Build history of the part. All positions in model axes, mm. A direction names the side the tool comes from. Round coordinates to 2 decimals unless told otherwise and drop trailing zeros. Order: outer loops, then holes, each group sorted by start corner. A loop starts at its lowest first (then second) coordinate and runs counter-clockwise, first axis right, second up. Notation, with made-up numbers: (21.5, 6) -> (47.5, 6) arc R9 cw to (47.5, 12) -> close; hole circle Ø6 at (31.25, 25.25). An arc over 180 degrees is marked (long way). Use a Markdown table: item, result. Add a question column.
Item 1: Two-plate mould, pull along X, no slides. Class faces 1 (the face through (59, 25, 18)), 2 (the face through (0, 0, 29)), 3 (the face through (69.14, 24.65, -29.1)): released by +X, released by -X, zero draft, split by the parting line, or undercut.
Item 2: Probe L1, parallel to Z at x = 42.5, y = 31; L2, parallel to X at y = 13.5, z = -10.5; L3, parallel to X at y = 19, z = -24. List the from-to ranges inside material, lowest first.
Item 3: Slice it at C-C, the plane z = -0.5. Give the cut face in (x, y), plus the area to 3 significant figures.
Item 4: Slice it at A-A, the plane x = 21. Give the cut face in (y, z).
Item 5: Slice it at B-B, the plane x = -60. Give the cut face in (y, z).
Item 6: 3-axis set-ups, long thin cutter, end or side, ignore diameter. For faces 4 (the face through (69.26, 15.726, 2.059)), 5 (the face through (67.74, 11.82, -2.93)), 6 (the face through (-60, 25, 18)): which of +Z, -Z, +X, -X, +Y, -Y reach the whole face in a straight line?
Item 7: Slice it at D-D, the plane y = 25. State how many separate pieces and enclosed holes the cut face has, plus the area to 3 significant figures.
from build123d import *

# Parameters (mm, degrees)
SKETCH1_R           = 2.75
SKETCH1_W           = 130
SKETCH1_H           = 38
BOSS_EXTRUDE1_DEPTH = 10
SKETCH1_2_W         = 130
SKETCH1_2_H         = 38
BOSS_EXTRUDE2_DEPTH = 10
SKETCH14_W          = 15
SKETCH14_H          = 36
SKETCH14_W_2        = 104
SKETCH14_H_2        = 9
CUT_EXTRUDE2_DEPTH  = 77.811457479
FILLET2_R           = 4
SKETCH15_R          = 2.75
BOSS_EXTRUDE3_DEPTH = 40
CUT_EXTRUDE3_REACH  = 153.658
SKETCH16_R          = 9.5
SKETCH17_R          = 13.5
CUT_EXTRUDE4_DEPTH  = 1.5


with BuildPart() as part:
    # Sketch1 → Boss-Extrude1 (new body)
    with BuildSketch(Plane(origin=(0, 0, 0), x_dir=(1, 0, 0), z_dir=(0, 1, 0))):
        with BuildLine():
            Line((67, 30), (-67, 30))
            ThreePointArc((-67, 30), (-69.121320344, 29.121320344), (-70, 27))
            Line((-70, 27), (-70, -27))
            ThreePointArc((-70, -27), (-69.121320344, -29.121320344), (-67, -30))
            Line((-67, -30), (67, -30))
            ThreePointArc((67, -30), (69.121320344, -29.121320344), (70, -27))
            Line((70, -27), (70, 27))
            ThreePointArc((70, 27), (69.121320344, 29.121320344), (67, 30))
        make_face()
        with Locations(Location((-60, 24, 0), (0, 0, 270))):
            Circle(SKETCH1_R, mode=Mode.SUBTRACT)
        with Locations(Location((-60, -24, 0), (0, 0, 270))):
            Circle(SKETCH1_R, mode=Mode.SUBTRACT)
        with Locations(Location((60, -24, 0), (0, 0, 270))):
            Circle(SKETCH1_R, mode=Mode.SUBTRACT)
        with Locations(Location((60, 24, 0), (0, 0, 270))):
            Circle(SKETCH1_R, mode=Mode.SUBTRACT)
        Rectangle(SKETCH1_W, SKETCH1_H, mode=Mode.SUBTRACT)
    extrude(amount=BOSS_EXTRUDE1_DEPTH)

    # Sketch1<2> → Boss-Extrude2 (add)
    with BuildSketch(Plane(origin=(0, 0, 0), x_dir=(1, 0, 0), z_dir=(0, 1, 0))):
        Rectangle(SKETCH1_2_W, SKETCH1_2_H)
    extrude(amount=BOSS_EXTRUDE2_DEPTH)

    # Sketch14 → Cut-Extrude2 (cut, through all)
    with BuildSketch(Plane(origin=(0, 10, 0), x_dir=(1, 0, 0), z_dir=(0, 1, 0))):
        with Locations((-59.5, 0)):
            Rectangle(SKETCH14_W, SKETCH14_H)
        Rectangle(SKETCH14_W_2, SKETCH14_H)
        with Locations((0, 22.5)):
            Rectangle(SKETCH14_W_2, SKETCH14_H_2)
        with Locations((59.5, 0)):
            Rectangle(SKETCH14_W, SKETCH14_H)
        with Locations((0, -22.5)):
            Rectangle(SKETCH14_W_2, SKETCH14_H_2)
    extrude(amount=-CUT_EXTRUDE2_DEPTH, mode=Mode.SUBTRACT)

    # Fillet2
    fillet2_edges = [part.edges().sort_by_distance(p)[0] for p in [
        (-67, 5, 18),
        (-67, 5, -18),
        (-52, 5, -18),
        (-52, 5, -27),
        (52, 5, -27),
        (52, 5, -18),
        (67, 5, -18),
        (67, 5, 18),
        (52, 5, 18),
        (52, 5, 27),
        (-52, 5, 27),
        (-52, 5, 18),
    ]]
    fillet(fillet2_edges, radius=FILLET2_R)

    # Sketch15 → Boss-Extrude3 (add)
    with BuildSketch(Plane(origin=(0, 10, 0), x_dir=(1, 0, 0), z_dir=(0, 1, 0))):
        with BuildLine():
            Line((67, 30), (-67, 30))
            ThreePointArc((-67, 30), (-69.121320344, 29.121320344), (-70, 27))
            Line((-70, 27), (-70, -27))
            ThreePointArc((-70, -27), (-69.121320344, -29.121320344), (-67, -30))
            Line((-67, -30), (67, -30))
            ThreePointArc((67, -30), (69.121320344, -29.121320344), (70, -27))
            Line((70, -27), (70, 27))
            ThreePointArc((70, 27), (69.121320344, 29.121320344), (67, 30))
        make_face()
        with Locations(Location((-60, 24, 0), (0, 0, 270))):
            Circle(SKETCH15_R, mode=Mode.SUBTRACT)
        with Locations(Location((-60, -24, 0), (0, 0, 270))):
            Circle(SKETCH15_R, mode=Mode.SUBTRACT)
        with Locations(Location((60, -24, 0), (0, 0, 270))):
            Circle(SKETCH15_R, mode=Mode.SUBTRACT)
        with Locations(Location((60, 24, 0), (0, 0, 270))):
            Circle(SKETCH15_R, mode=Mode.SUBTRACT)
        with BuildLine():
            Line((56, -18), (63, -18))
            ThreePointArc((63, -18), (65.828427125, -16.828427125), (67, -14))
            Line((67, -14), (67, 14))
            ThreePointArc((67, 14), (65.828427125, 16.828427125), (63, 18))
            Line((63, 18), (56, 18))
            ThreePointArc((56, 18), (53.171572875, 19.171572875), (52, 22))
            Line((52, 22), (52, 23))
            ThreePointArc((52, 23), (50.828427125, 25.828427125), (48, 27))
            Line((48, 27), (-48, 27))
            ThreePointArc((-48, 27), (-50.828427125, 25.828427125), (-52, 23))
            Line((-52, 23), (-52, 22))
            ThreePointArc((-52, 22), (-53.171572875, 19.171572875), (-56, 18))
            Line((-56, 18), (-63, 18))
            ThreePointArc((-63, 18), (-65.828427125, 16.828427125), (-67, 14))
            Line((-67, 14), (-67, -14))
            ThreePointArc((-67, -14), (-65.828427125, -16.828427125), (-63, -18))
            Line((-63, -18), (-56, -18))
            ThreePointArc((-56, -18), (-53.171572875, -19.171572875), (-52, -22))
            Line((-52, -22), (-52, -23))
            ThreePointArc((-52, -23), (-50.828427125, -25.828427125), (-48, -27))
            Line((-48, -27), (48, -27))
            ThreePointArc((48, -27), (50.828427125, -25.828427125), (52, -23))
            Line((52, -23), (52, -22))
            ThreePointArc((52, -22), (53.171572875, -19.171572875), (56, -18))
        make_face(mode=Mode.SUBTRACT)
    extrude(amount=BOSS_EXTRUDE3_DEPTH)

    # Sketch16 → Cut-Extrude3 (cut, up to next)
    with BuildSketch(Plane(origin=(70, 0, 0), x_dir=(0, 0, -1), z_dir=(1, 0, 0)), mode=Mode.PRIVATE) as cut_extrude3_sk1:
        with Locations((0, 25)):
            Circle(SKETCH16_R)
    cut_extrude3_tool1 = extrude(cut_extrude3_sk1.sketch, amount=-CUT_EXTRUDE3_REACH, mode=Mode.PRIVATE) & part.part
    add(cut_extrude3_tool1.solids().sort_by_distance((70, 25, 0))[0], mode=Mode.SUBTRACT)

    # Sketch17 → Cut-Extrude4 (cut)
    with BuildSketch(Plane.ZY.offset(-67)):
        with Locations((0, 25)):
            Circle(SKETCH17_R)
    extrude(amount=-CUT_EXTRUDE4_DEPTH, mode=Mode.SUBTRACT)


solid = part.part
Check sheet entries:
| question | item | result |
|---|---|---|
| 1 | face 1 | undercut |
| 1 | face 2 | zero draft |
| 1 | face 3 | released by +X |
| 2 | L1 | -30 to -27, 27 to 30 |
| 2 | L2 | -70 to -67, 67 to 70 |
| 2 | L3 | -70 to -62.75, -57.25 to -51.87, 51.87 to 57.25, 62.75 to 70 |
| 3 | outline | (-70, 0) -> (-67, 0) -> (-67, 50) -> (-70, 50) -> close; (67, 0) -> (70, 0) -> (70, 15.51) -> (68.5, 15.51) -> (68.5, 11.51) -> (67, 11.51) -> close; (67, 38.49) -> (68.5, 38.49) -> (68.5, 34.49) -> (70, 34.49) -> (70, 50) -> (67, 50) -> close |
| 3 | area | 231 mm2 |
| 4 | outline | (0, -30) -> (50, -30) -> (50, -27) -> (0, -27) -> close; (0, 27) -> (50, 27) -> (50, 30) -> (0, 30) -> close |
| 5 | outline | (0, -30) -> (50, -30) -> (50, -26.75) -> (0, -26.75) -> close; (0, -21.25) -> (50, -21.25) -> (50, -18) -> (0, -18) -> close; (0, 18) -> (50, 18) -> (50, 21.25) -> (0, 21.25) -> close; (0, 26.75) -> (50, 26.75) -> (50, 30) -> (0, 30) -> close |
| 6 | face 4 | +X |
| 6 | face 5 | none |
| 6 | face 6 | +Y, -Y |
| 7 | separate pieces | 1 |
| 7 | enclosed holes | 4 |
| 7 | area | 1,550 mm2 |
